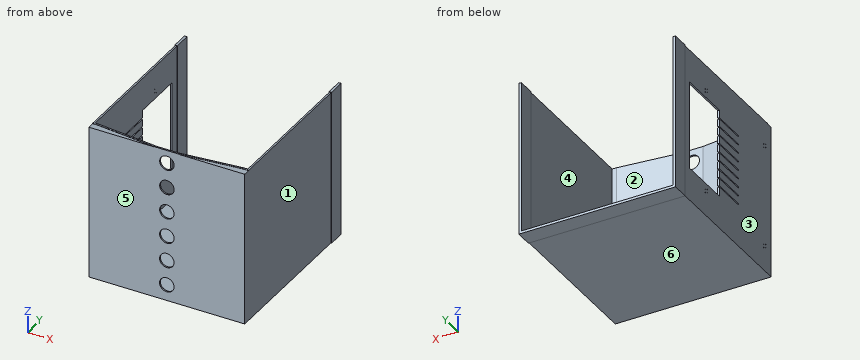
```python
from build123d import *

# Parameters (mm, degrees)
SKETCH1_W           = 914.4
SKETCH1_H           = 914.4
BOSS_EXTRUDE1_DEPTH = 50
SKETCH2_W           = 914.4
SKETCH2_H           = 914.4
BOSS_EXTRUDE2_DEPTH = 10
SKETCH4_W           = 914.4
SKETCH4_H           = 914.4
BOSS_EXTRUDE3_DEPTH = 10
SKETCH5_W           = 934.4
SKETCH5_H           = 914.4
BOSS_EXTRUDE4_DEPTH = 10
CUT_EXTRUDE2_DEPTH  = 925.4
BOSS_EXTRUDE5_DEPTH = 10
SKETCH10_R          = 43.356897361
CUT_EXTRUDE3_DEPTH  = 10.220124983
SKETCH11_W          = 530.7
SKETCH11_H          = 315.6
CUT_EXTRUDE4_DEPTH  = 10
BOSS_EXTRUDE7_DEPTH = 101.6
BOSS_EXTRUDE8_DEPTH = 922.782
SKETCH17_R          = 2.5
CUT_EXTRUDE5_DEPTH  = 10
SKETCH18_W          = 7.62
SKETCH18_H          = 203.2
CUT_EXTRUDE6_DEPTH  = 10


with BuildPart() as part:
    # Sketch1 → Boss-Extrude1 (new body)
    with BuildSketch(Plane(origin=(0, 0, 0), x_dir=(1, 0, 0), z_dir=(0, 1, 0))):
        with Locations((2.50749543, -165.494698355)):
            Rectangle(SKETCH1_W, SKETCH1_H)
    extrude(amount=BOSS_EXTRUDE1_DEPTH)

    # Sketch2 → Boss-Extrude2 (add)
    with BuildSketch(Plane(origin=(459.70749543, 0, 0), x_dir=(0, 0, -1), z_dir=(1, 0, 0))):
        with Locations((-165.494698355, 457.2)):
            Rectangle(SKETCH2_W, SKETCH2_H)
    extrude(amount=BOSS_EXTRUDE2_DEPTH)

    # Sketch4 → Boss-Extrude3 (add)
    with BuildSketch(Plane.ZY.offset(454.69250457)):
        with Locations((165.494698355, 457.2)):
            Rectangle(SKETCH4_W, SKETCH4_H)
    extrude(amount=BOSS_EXTRUDE3_DEPTH)

    # Sketch5 → Boss-Extrude4 (add)
    with BuildSketch(Plane(origin=(0, 0, -291.705301645), x_dir=(-1, 0, 0), z_dir=(0, 0, -1))):
        with Locations((-2.50749543, 457.2)):
            Rectangle(SKETCH5_W, SKETCH5_H)
    extrude(amount=BOSS_EXTRUDE4_DEPTH)

    # Sketch6 → Cut-Extrude2 (cut, through all)
    with BuildSketch(Plane.XY.offset(622.694698355)):
        Polygon((-464.69250457, 0), (-61.618954828, 0), (-439.884510812, 40), (-464.69250457, 40), align=None)
        Polygon((-439.884510812, 50), (-61.618954828, 9.220124983), (68.644680345, 9.220124983), (434.384886793, 50), align=None)
        Polygon((434.384886793, 40), (68.644680345, 0), (469.70749543, 0), (469.70749543, 40), align=None)
    extrude(amount=-CUT_EXTRUDE2_DEPTH, mode=Mode.SUBTRACT)

    # Sketch8 → Boss-Extrude5 (add)
    with BuildSketch(Plane(origin=(0, 0, -301.705301645), x_dir=(-1, 0, 0), z_dir=(0, 0, -1))):
        Polygon((-434.384886793, 50), (-68.644680345, 9.220124983), (61.618954828, 9.220124983), (439.884510812, 50), align=None)
    extrude(amount=-BOSS_EXTRUDE5_DEPTH)

    # Sketch10 → Cut-Extrude3 (cut, through all)
    with BuildSketch(Plane(origin=(0, 9.220124983, 0), x_dir=(1, 0, 0), z_dir=(0, 1, 0))):
        with Locations((3.426978674, -544.581550471)):
            Circle(SKETCH10_R)
        with Locations((3.262056312, -394.581641136)):
            Circle(SKETCH10_R)
        with Locations((3.097133949, -244.5817318)):
            Circle(SKETCH10_R)
        with Locations((2.932211587, -94.581822465)):
            Circle(SKETCH10_R)
        with Locations((2.767289224, 55.41808687)):
            Circle(SKETCH10_R)
        with Locations((2.602366862, 205.417996206)):
            Circle(SKETCH10_R)
    extrude(amount=-CUT_EXTRUDE3_DEPTH, mode=Mode.SUBTRACT)

    # Sketch11 → Cut-Extrude4 (cut)
    with BuildSketch(Plane.ZY.offset(464.69250457)):
        with Locations((160.494698355, 705.8)):
            Rectangle(SKETCH11_W, SKETCH11_H)
    extrude(amount=-CUT_EXTRUDE4_DEPTH, mode=Mode.SUBTRACT)

    # Sketch14 → Boss-Extrude7 (add)
    with BuildSketch(Plane(origin=(0, 914.4, 0), x_dir=(1, 0, 0), z_dir=(0, 1, 0))):
        Polygon((457.16749543, 289.165301645), (457.16749543, -625.234698355), (472.24749543, -625.234698355), (472.24749543, 304.245301645), (-467.23250457, 304.245301645), (-467.23250457, -625.234698355), (-452.15250457, -625.234698355), (-452.15250457, 289.165301645), align=None)
    extrude(amount=BOSS_EXTRUDE7_DEPTH)

    # Sketch16 → Boss-Extrude8 (add)
    with BuildSketch(Plane(origin=(0, 0, -301.705301645), x_dir=(-1, 0, 0), z_dir=(0, 0, -1))):
        Polygon((-469.70749543, 40), (-469.70749543, 0), (-68.644680345, 0), (-434.384886793, 40), align=None)
        Polygon((61.618954828, 0), (439.884510812, 40), (464.69250457, 40), (464.69250457, 0), align=None)
    extrude(amount=-BOSS_EXTRUDE8_DEPTH)

    # Sketch17 → Cut-Extrude5 (cut)
    with BuildSketch(Plane.ZY.offset(464.69250457)):
        with Locations((-164.105301645, 77.736709547)):
            Circle(SKETCH17_R)
        with Locations((-144.105301645, 77.736709547)):
            Circle(SKETCH17_R)
        with Locations((-134.105301645, 57.736709547)):
            Circle(SKETCH17_R)
        with Locations((-154.105301645, 57.736709547)):
            Circle(SKETCH17_R)
        with Locations((474.694698355, 77.736709547)):
            Circle(SKETCH17_R)
        with Locations((484.694698355, 57.736709547)):
            Circle(SKETCH17_R)
        with Locations((464.694698355, 57.736709547)):
            Circle(SKETCH17_R)
        with Locations((454.694698355, 77.736709547)):
            Circle(SKETCH17_R)
        with Locations((-164.105301645, 698.149833047)):
            Circle(SKETCH17_R)
        with Locations((-144.105301645, 698.149833047)):
            Circle(SKETCH17_R)
        with Locations((-134.105301645, 678.149833047)):
            Circle(SKETCH17_R)
        with Locations((-154.105301645, 678.149833047)):
            Circle(SKETCH17_R)
        with Locations((474.694698355, 698.149833047)):
            Circle(SKETCH17_R)
        with Locations((484.694698355, 678.149833047)):
            Circle(SKETCH17_R)
        with Locations((464.694698355, 678.149833047)):
            Circle(SKETCH17_R)
        with Locations((454.694698355, 698.149833047)):
            Circle(SKETCH17_R)
    extrude(amount=-CUT_EXTRUDE5_DEPTH, mode=Mode.SUBTRACT)

    # Sketch18 → Cut-Extrude6 (cut)
    with BuildSketch(Plane.ZY.offset(464.69250457)):
        with Locations((-43.895301645, 446.4)):
            Rectangle(SKETCH18_W, SKETCH18_H)
        with Locations((8.174698355, 446.4)):
            Rectangle(SKETCH18_W, SKETCH18_H)
        with Locations((60.244698355, 446.4)):
            Rectangle(SKETCH18_W, SKETCH18_H)
        with Locations((113.584698355, 446.4)):
            Rectangle(SKETCH18_W, SKETCH18_H)
        with Locations((165.654698355, 446.4)):
            Rectangle(SKETCH18_W, SKETCH18_H)
        with Locations((217.724698355, 446.4)):
            Rectangle(SKETCH18_W, SKETCH18_H)
        with Locations((271.064698355, 446.4)):
            Rectangle(SKETCH18_W, SKETCH18_H)
        with Locations((323.134698355, 446.4)):
            Rectangle(SKETCH18_W, SKETCH18_H)
        with Locations((375.204698355, 446.4)):
            Rectangle(SKETCH18_W, SKETCH18_H)
    extrude(amount=-CUT_EXTRUDE6_DEPTH, mode=Mode.SUBTRACT)


solid = part.part
```
Could you check a few things on this model? Use its own coordinates, in mm. Face numbers are marked on the shaded views. A direction names the side the tool comes from. Round coordinates to 2 decimals unless told otherwise and drop trailing zeros. Loops run counter-clockwise (first coordinate to the right, second up) from the corner with the lowest first, then second, coordinate; pieces in that order, holes last. Notation, with made-up numbers: (3, 23.5) - (41, 23.5) arc R25 ccw to (41, 59.5) - close; hole circle Ø2 at (41.5, -36). An arc over 180 degrees is marked (long way). Answer in a Markdown table with one row per item. Add a question column.
(1) If we mould it in two halves opening along X, with no side actions, what happens to the marked faces 1, 2 and 3? For each: pulls with the +X half, pulls with the -X half, needs draft (parallel to the pull), parting line crosses it, or undercut.
(2) If we section it at B-B (y = 157): Please give me the cut outline in (x, z).
(3) For the marked faces 4, 5 and 6, which set-ups out of +Z, -Z, +X, -X, +Y, -Y let a thin tool reach every point of the face, with its end or its side?
(4) I need wall thicknesses on line 1 along X through (y, z) = (445, -39); line 2 along Z through (x, y) = (388, 293); line 3 along X through (y, z) = (558, 418.5). Which ranges of each line are inside material? Lowest first, please.
(5) If we section it at D-D (x = 130.5): Please give me the cut outline in (y, z), plus the area to 3 significant figures.
(6) I'm going to push flat-ended pins straight in: pin 1 (6 mm diameter, centred on y = 698.15, z = 454.69, fed in from -X); pin 2 (10 mm diameter, centred on y = 563.5, z = 524, fed in from +X); pin 3 (3 mm diameter, centred on x = -461.5, y = 749, fed in from -Z). Where does each tip first touch, or does it pass through?
(7) If we section it at A-A (x = -10): State how many separate pieces and enclosed holes the cut face has, plus the area to 3 significant figures.
Model answer:
| question | item | result |
|---|---|---|
| 1 | face 1 | pulls with the +X half |
| 1 | face 2 | undercut |
| 1 | face 3 | pulls with the -X half |
| 2 | outline | (-464.69, -301.71) - (469.71, -301.71) - (469.71, 622.69) - (459.71, 622.69) - (459.71, -291.71) - (-454.69, -291.71) - (-454.69, 622.69) - (-464.69, 622.69) - close |
| 3 | face 4 | +Z |
| 3 | face 5 | +Z, -Z, +X, -X, -Y |
| 3 | face 6 | -Z, +X, -X, -Y |
| 4 | line 1 | x = -464.69 to -454.69, 459.71 to 469.71 |
| 4 | line 2 | z = -301.71 to -291.71 |
| 4 | line 3 | x = 459.71 to 469.71 |
| 5 | outline | (0, -301.71) - (914.4, -301.71) - (914.4, -304.25) - (1016, -304.25) - (1016, -289.17) - (914.4, -289.17) - (914.4, -291.71) - (16.12, -291.71) - (16.12, 622.69) - (6.76, 622.69) - (6.76, 621.08) - (0, 621.08) - close |
| 5 | area | 25,400 mm² |
| 6 | pin 1 | stops at x = -464.69 |
| 6 | pin 2 | stops at x = 469.71 |
| 6 | pin 3 | stops at z = -301.71 |
| 7 | separate pieces | 7 |
| 7 | enclosed holes | 0 |
| 7 | area | 14,500 mm² |
